The listing builds one solid part. Answer for the finished solid, in the listing's coordinates (mm). A direction names the side the tool comes from. Give positions to 0.01 mm unless a question says otherwise; leave off trailing zeros. Write each loop counter-clockwise with the first axis right and the second up, starting at its lowest first coordinate (ties: lowest second). Pieces come first, ordered by that corner, then holes. Notation, with made-up numbers: (-20.75, 73.25) - (14.25, 73.25) arc R34 cw to (14.25, 111.25) - close; hole circle Ø9 at (6.5, 73.25). An arc over 180 degrees is marked (long way). Answer as CSV lines item,"result". Start each with the question number.
(1) Find section D-D (y = 8). Write down the section's boundary in (x, z).
(2) For faces 4 (the face through (0, 8, 5.9)), 5 (the face through (-8, 0, 2)), 6 (the face through (1.124, -1.799, 0.567)), 7 (the face through (2, 0, 0)), determine the directions among +Z, -Z, +X, -X, +Y, -Y from which every point of the face is accessible in a straight line to the end or side of a thin tool.
(3) For a pull along Z with two mould halves and no side action, classify faces 1 (the face through (-2, -10, 8)), 2 (the face through (0.1, 5.5, 7.5)), 3 (the face through (0, 8, 20)) as pulls with the +Z half, pulls with the -Z half, needs draft (parallel to the pull), parting line crosses it, or undercut.
(4) Find section A-A (y = 0). Write down the section's boundary in (x, z).
(5) Find section C-C (z = 8.25). Write down the section's boundary in (x, y), then the cut area to 3 significant figures.
(6) Find section B-B (x = 0). Write down the section's boundary in (y, z), then the cut area to 3 significant figures.
(7) Each of these flat-tipped pins is pushed along its axis until it touches: pin 1 Ø2.5 at (x, y) = (6.5, 2) entering from +Z; pin 2 Ø4.5 at (x, y) = (0, 0) entering from +Z; pin 3 Ø1 at (x, y) = (-4.5, -4.5) entering from +Z. Where does it stop, or does it pass through?
(8) Straight lines are drawn through the part: probe 1 along Y at (x, z) = (0, 0.4); probe 2 along Y at (x, z) = (-1.5, 7.25); probe 3 along X at (y, z) = (5.65, 10). For each, find the intervals that lie inside material, in ascending order.
from build123d import *

# Parameters (mm, degrees)
SZKIC1_W                    = 20
SZKIC1_H                    = 20
DODANIE_WYCI_GNI_CIE1_DEPTH = 2
SZKIC2_R                    = 1.75
WYTNIJ_WYCI_GNI_CIE1_DEPTH  = 15.282856857
SZKIC3_W                    = 20
SZKIC3_H                    = 5
SZKIC3_H_2                  = 4
DODANIE_WYCI_GNI_CIE2_DEPTH = 18
SZKIC4_R                    = 2.5
WYTNIJ_WYCI_GNI_CIE2_DEPTH  = 31
WYTNIJ_WYCI_GNI_CIE3_DEPTH  = 4
WYTNIJ_WYCI_GNI_CIE5_START  = -4
SZKIC7_R                    = 9.5
WYTNIJ_WYCI_GNI_CIE5_DEPTH  = 11


with BuildPart() as part:
    # Szkic1 → Dodanie-wyciągnięcie1 (new body)
    with BuildSketch(Plane.XY):
        Rectangle(SZKIC1_W, SZKIC1_H)
    extrude(amount=DODANIE_WYCI_GNI_CIE1_DEPTH)

    # Szkic2 → Wytnij-wyciągnięcie1 (cut, through all)
    with BuildSketch(Plane.XY.offset(2)):
        Circle(SZKIC2_R)
    extrude(amount=-WYTNIJ_WYCI_GNI_CIE1_DEPTH, mode=Mode.SUBTRACT)

    # Szkic3 → Dodanie-wyciągnięcie2 (add)
    with BuildSketch(Plane.XY.offset(2)):
        with Locations((0, 7.5)):
            Rectangle(SZKIC3_W, SZKIC3_H)
        with Locations((0, -8)):
            Rectangle(SZKIC3_W, SZKIC3_H_2)
    extrude(amount=DODANIE_WYCI_GNI_CIE2_DEPTH)

    # Szkic4 → Wytnij-wyciągnięcie2 (cut, through all)
    with BuildSketch(Plane(origin=(0, 10, 0), x_dir=(1, 0, 0), z_dir=(0, 1, 0))):
        with Locations(Location((0, -10, 0), (0, 0, 270))):
            Circle(SZKIC4_R)
    extrude(amount=-WYTNIJ_WYCI_GNI_CIE2_DEPTH, mode=Mode.SUBTRACT)

    # Szkic6 → Wytnij-wyciągnięcie3 (cut)
    with BuildSketch(Plane(origin=(0, 10, 0), x_dir=(1, 0, 0), z_dir=(0, 1, 0))):
        Polygon((4.734272207, -10), (2.367136104, -5.9), (-2.367136104, -5.9), (-4.734272207, -10), (-2.367136104, -14.1), (2.367136104, -14.1), align=None)
    extrude(amount=-WYTNIJ_WYCI_GNI_CIE3_DEPTH, mode=Mode.SUBTRACT)

    # Szkic7 → Wytnij-wyciągnięcie5 (cut)
    with BuildSketch(Plane.XZ.offset(10).offset(WYTNIJ_WYCI_GNI_CIE5_START)):
        with Locations((0, 10)):
            Circle(SZKIC7_R)
    extrude(amount=-WYTNIJ_WYCI_GNI_CIE5_DEPTH, mode=Mode.SUBTRACT)


solid = part.part
Result set:
1,outline,"(-10, 0) - (10, 0) - (10, 20) - (-10, 20) - close; hole (-4.73, 10) - (-2.37, 5.9) - (2.37, 5.9) - (4.73, 10) - (2.37, 14.1) - (-2.37, 14.1) - close"
2,face 4,"+Y"
2,face 5,"+Z, +X, -X"
2,face 6,"+Z"
2,face 7,"-Z, +X, -X, +Y, -Y"
3,face 1,"needs draft"
3,face 2,"undercut"
3,face 3,"pulls with the +Z half"
4,outline,"(-10, 0) - (-1.75, 0) - (-1.75, 0.66) arc R9.5 cw to (-5.12, 2) - (-10, 2) - close; (1.75, 0) - (10, 0) - (10, 2) - (5.12, 2) arc R9.5 cw to (1.75, 0.66) - close"
5,outline,"(-10, -10) - (-1.79, -10) - (-1.79, -6) - (-10, -6) - close; (-10, 5) - (-1.79, 5) - (-1.79, 6) - (-3.72, 6) - (-3.72, 10) - (-10, 10) - close; (1.79, -10) - (10, -10) - (10, -6) - (1.79, -6) - close; (1.79, 5) - (10, 5) - (10, 10) - (3.72, 10) - (3.72, 6) - (1.79, 6) - close"
5,area,"132 mm^2"
6,outline,"(-10, 0) - (-1.75, 0) - (-1.75, 0.5) - (-6, 0.5) - (-6, 7.5) - (-10, 7.5) - close; (-10, 12.5) - (-6, 12.5) - (-6, 20) - (-10, 20) - close; (1.75, 0) - (10, 0) - (10, 5.9) - (6, 5.9) - (6, 7.5) - (5, 7.5) - (5, 0.5) - (1.75, 0.5) - close; (5, 12.5) - (6, 12.5) - (6, 14.1) - (10, 14.1) - (10, 20) - (5, 20) - close"
6,area,"126 mm^2"
7,pin 1,"z = 2"
7,pin 2,"z = 0.77"
7,pin 3,"z = 1.92"
8,probe 1,"-10 to -1.75, 1.75 to 10"
8,probe 2,"-10 to -6, 5 to 6"
8,probe 3,"-10 to -2.5, 2.5 to 10"
